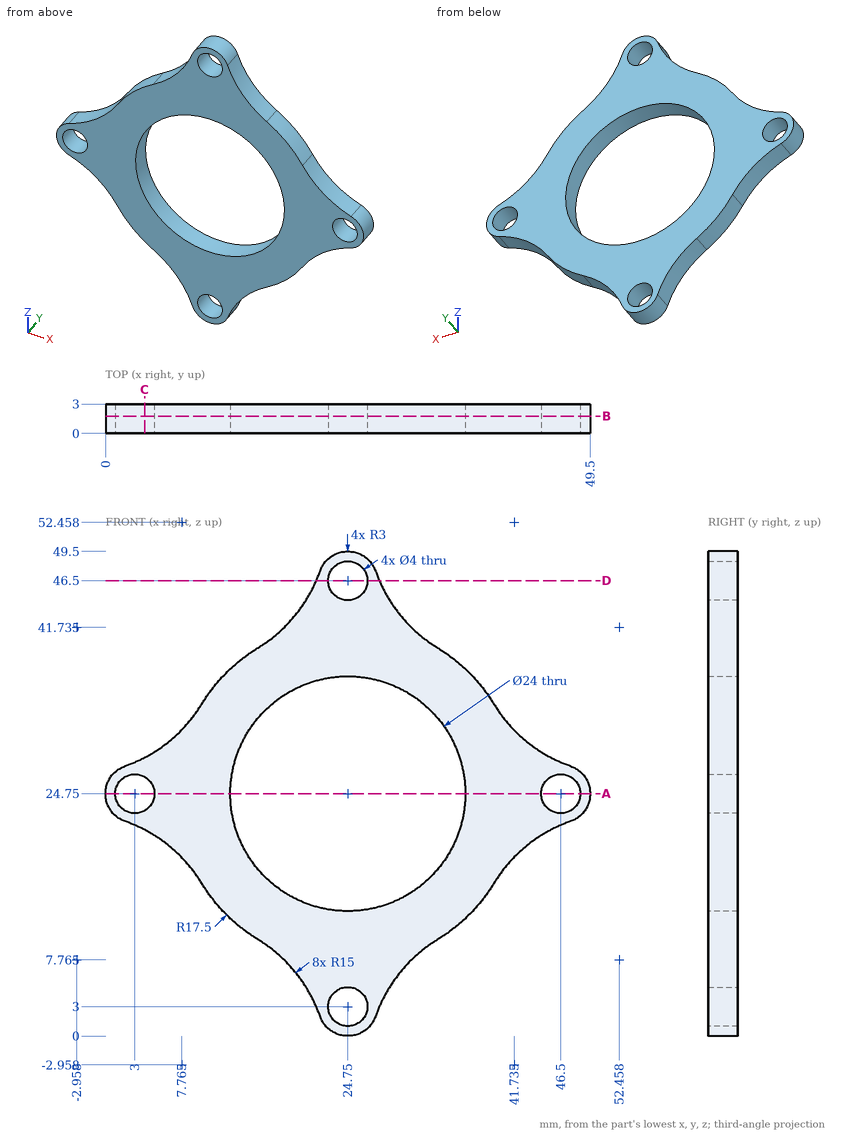
Design review of the part shown in the three views and the two pictorial views. Dimensions are in mm from the part's minimum x, y and z. Round coordinates to 2 decimals unless told otherwise and drop trailing zeros. Loops run counter-clockwise (first coordinate to the right, second up) from the corner with the lowest first, then second, coordinate; pieces in that order, holes last. Notation, with made-up numbers: (-15, 22.25) -> (13, 22.25) arc R24 ccw to (13, 41.25) -> close; hole circle Ø3 at (35.5, 63). An arc over 180 degrees is marked (long way). Answer as a JSON object with one key per item and string values. Group by question number.
1) We need section D-D on z = 46.5. Write out the cut boundary in (x, y).
2) For pin 1 Ø1 at (y, z) = (1, 19) entering from +X (1 decimal); pin 2 Ø1 at (x, y) = (27, 2) entering from +Z, all flat-tipped, find the tip position at first contact; note any pin that passes through.
3) We need section B-B on y = 1.75. Give the number of separate pieces and of enclosed holes in the cut face, then the cut area to 3 significant figures.
4) We need section A-A on z = 24.75. Write out the cut boundary in (x, y), then the cut area to 3 significant figures.
5) We need section C-C on x = 4. Write out the cut boundary in (y, z), then the cut area to 3 significant figures.
6) For line 1 (X direction, y = 1.2, z = 24.75); line 2 (Z direction, x = 23, y = 2.85) (1 decimal); line 3 (Z direction, x = 17.5, y = 0.4) (1 decimal), list the stretches that pass through material, from the lowest coordinate up. Write a range as [from, to].
Result set:
{
 "1": {"outline": "(21.53, 0) -> (22.75, 0) -> (22.75, 3) -> (21.53, 3) -> close; (26.75, 0) -> (27.97, 0) -> (27.97, 3) -> (26.75, 3) -> close"},
 "2": {"pin 1": "x = 43.1", "pin 2": "z = 48.94"},
 "3": {"separate pieces": "1", "enclosed holes": "5", "area": "693 mm²"},
 "4": {"outline": "(0, 0) -> (1, 0) -> (1, 3) -> (0, 3) -> close; (5, 0) -> (12.75, 0) -> (12.75, 3) -> (5, 3) -> close; (36.75, 0) -> (44.5, 0) -> (44.5, 3) -> (36.75, 3) -> close; (48.5, 0) -> (49.5, 0) -> (49.5, 3) -> (48.5, 3) -> close", "area": "52.5 mm²"},
 "5": {"outline": "(0, 21.05) -> (3, 21.05) -> (3, 23.02) -> (0, 23.02) -> close; (0, 26.48) -> (3, 26.48) -> (3, 28.45) -> (0, 28.45) -> close", "area": "11.8 mm²"},
 "6": {"line 1": "[0, 1], [5, 12.75], [36.75, 44.5], [48.5, 49.5]", "line 2": "[0.6, 2], [4, 12.9], [36.6, 45.5], [47.5, 48.9]", "line 3": "[8.5, 15.2], [34.3, 41]"}
}
